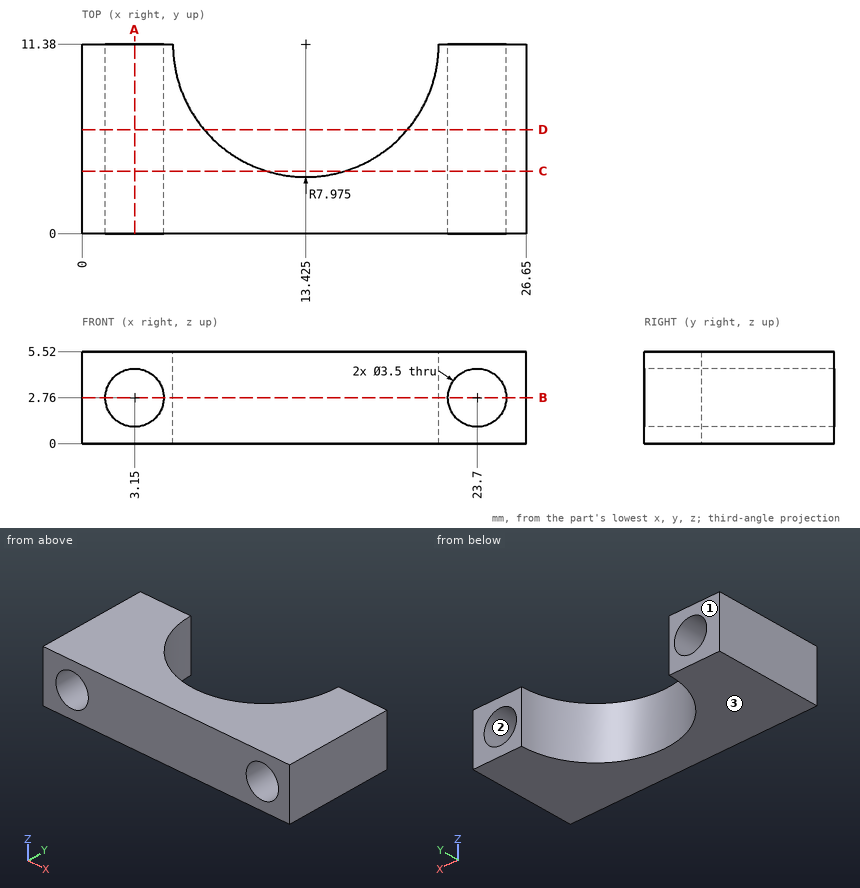
Study the drawing (mm; zero at the part's minimum x, y, z) and answer. Round coordinates to 2 decimals unless told otherwise and drop trailing zeros. Write each loop counter-clockwise with the first axis right and the second up, starting at its lowest first coordinate (ties: lowest second). Pieces come first, ordered by that corner, then holes. Notation, with made-up numbers: (41.5, 77) -> (57.5, 77) arc R21 ccw to (57.5, 98) -> close; hole circle Ø5 at (67.25, 7). An arc over 180 degrees is marked (long way). Write item = value, one per line.
1) Section A-A on x = 3.15 is taken. Write down the section's boundary in (y, z).
Check values:
outline = (0, 0) -> (11.38, 0) -> (11.38, 1.01) -> (0, 1.01) -> close; (0, 4.51) -> (11.38, 4.51) -> (11.38, 5.52) -> (0, 5.52) -> close
2) Given pin 1 (3 mm diameter, centred on x = 3.15, z = 2.76, fed in from -Y), flat-ended and moving along its own axis, determine where the tip first touches the part or whether it passes through.
Check values:
pin_1 = through
3) Section B-B on z = 2.76 is taken. Write down the section's boundary in (x, y) (3 decimals), plus the area to 3 significant figures.
Check values:
outline = (0, 0) -> (1.4, 0) -> (1.4, 11.38) -> (0, 11.38) -> close; (4.9, 0) -> (21.95, 0) -> (21.95, 11.38) -> (21.4, 11.38) arc R7.975 cw to (5.45, 11.38) -> (4.9, 11.38) -> close; (25.45, 0) -> (26.65, 0) -> (26.65, 11.38) -> (25.45, 11.38) -> close
area = 124 mm²
4) Section C-C on y = 3.75 is taken. Write down the section's boundary in (x, z), plus the area to 3 significant figures.
Check values:
outline = (0, 0) -> (11.1, 0) -> (11.1, 5.52) -> (0, 5.52) -> close; (15.75, 0) -> (26.65, 0) -> (26.65, 5.52) -> (15.75, 5.52) -> close; hole circle Ø3.5 at (3.15, 2.76); hole circle Ø3.5 at (23.7, 2.76)
area = 102 mm²
5) Straight lines are drawn through the part: line 1 along X through (y, z) = (7, 1.5); line 2 along X through (y, z) = (8.25, 1.7); line 3 along X through (y, z) = (3, 1.6). For each, find the intervals that lie inside material, in ascending order. Write a range as [from, to].
Check values:
line_1 = [0, 1.94], [4.36, 6.76], [20.09, 22.49], [24.91, 26.65]
line_2 = [0, 1.76], [4.54, 6.09], [20.76, 22.31], [25.09, 26.65]
line_3 = [0, 1.84], [4.46, 22.39], [25.01, 26.65]
6) For a pull along Z with two mould halves and no side action, classify the marked faces 1, 2 and 3 as released by +Z, released by -Z, zero draft, split by the parting line, or undercut.
Check values:
face_1 = zero draft
face_2 = undercut
face_3 = released by -Z
7) Section D-D on y = 6.25 is taken. Write down the section's boundary in (x, z), plus the area to 3 significant figures.
Check values:
outline = (0, 0) -> (7.32, 0) -> (7.32, 5.52) -> (0, 5.52) -> close; (19.53, 0) -> (26.65, 0) -> (26.65, 5.52) -> (19.53, 5.52) -> close; hole circle Ø3.5 at (3.15, 2.76); hole circle Ø3.5 at (23.7, 2.76)
area = 60.5 mm²
